For this review, take the finished solid that the model builds, in its own axes (mm). Round coordinates to 2 decimals unless told otherwise and drop trailing zeros. Loops run counter-clockwise (first coordinate to the right, second up) from the corner with the lowest first, then second, coordinate; pieces in that order, holes last.
1) Take a section at A-A (y = 0). State the section outline as (x, z) points (3 decimals).
2) Insertion check: pin 1 (6 mm diameter, centred on x = 141.5, z = 7.5, fed in from +Y); pin 2 (2 mm diameter, centred on y = 79, z = 5.5, fed in from +X); pin 3 (1 mm diameter, centred on x = 88.5, z = 10, fed in from -Y). Each pin has a flat end and moves straight along its axis. Give the tip position at first contact, or say it passes through.
3) Take a section at B-B (x = 0). State the section outline as (y, z) points (3 decimals), then the cut area to 3 significant figures.
4) Take a section at C-C (z = 5.75). State the section outline as (x, y) points (3 decimals), then the cut area to 3 significant figures.
5) Wall thickness on L1, parallel to Y at x = 0, z = 8 (3 decimals); L2, parallel to Y at x = 108.5, z = 11.5; L3, parallel to Y at x = 12.5, z = 10.75: over which ranges is each line inside the solid? List them lowest first.
6) Take a section at D-D (x = 122). State the section outline as (y, z) points, then the cut area to 3 significant figures.
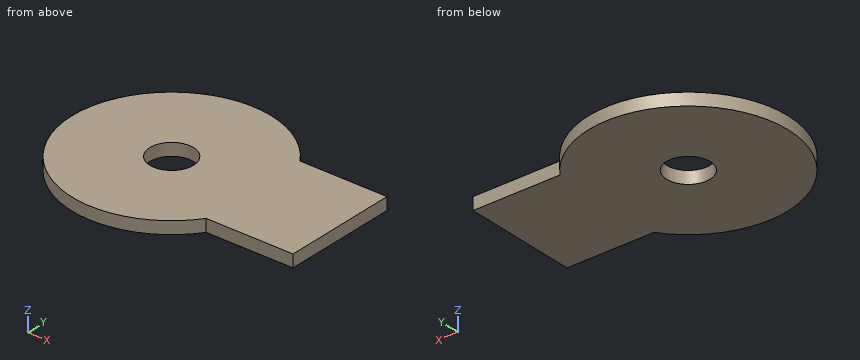
```python
from build123d import *

# Parameters (mm, degrees)
SKETCH1_R           = 101.6
SKETCH1_R_2         = 22.225
SKETCH1_W           = 88.659510459
SKETCH1_H           = 117.09666856
BOSS_EXTRUDE1_DEPTH = 12.7


with BuildPart() as part:
    # Sketch1 → Boss-Extrude1 (new body)
    with BuildSketch(Plane.XY):
        Circle(SKETCH1_R)
        Circle(SKETCH1_R_2, mode=Mode.SUBTRACT)
        with Locations((127.363799772, 0)):
            Rectangle(SKETCH1_W, SKETCH1_H)
    extrude(amount=BOSS_EXTRUDE1_DEPTH)


solid = part.part
```
Response:
1. outline: (-101.6, 0) - (-22.225, 0) - (-22.225, 12.7) - (-101.6, 12.7) - close; (22.225, 0) - (171.694, 0) - (171.694, 12.7) - (22.225, 12.7) - close
2. pin 1: stops at y = 58.55
2. pin 2: stops at x = 65.1
2. pin 3: stops at y = -58.55
3. outline: (-101.6, 0) - (-22.225, 0) - (-22.225, 12.7) - (-101.6, 12.7) - close; (22.225, 0) - (101.6, 0) - (101.6, 12.7) - (22.225, 12.7) - close
3. area: 2,020 mm2
4. outline: (83.034, -58.548) - (171.694, -58.548) - (171.694, 58.548) - (83.034, 58.548) arc R101.6 ccw (long way) to start; hole circle Ø44.45 at (0, 0)
4. area: 39,800 mm2
5. L1: y = -101.6 to -22.225, 22.225 to 101.6
5. L2: y = -58.55 to 58.55
5. L3: y = -100.83 to -18.38, 18.38 to 100.83
6. outline: (-58.55, 0) - (58.55, 0) - (58.55, 12.7) - (-58.55, 12.7) - close
6. area: 1,490 mm2
